The listing builds one solid part. Answer for the finished solid, in the listing's coordinates (mm). A direction names the side the tool comes from. Give positions to 0.01 mm unless a question says otherwise; leave off trailing zeros. Loops run counter-clockwise (first coordinate to the right, second up) from the corner with the lowest first, then second, coordinate; pieces in that order, holes last. Notation, with made-up numbers: M 82,68.5 L 124,68.5 A29 cw 124,88.5 Z; hole C 33,53 d1. An arc over 180 degrees is marked long. Use one line per item in the form item = value. Start each with the question number.
1. A straight line is drawn through the part: line 1 (X direction, y = -5.5, z = 11.5). Find the intervals that lie inside material, in ascending order. Write a range as from..to.
2. For faces 1 (the face through (0, -15, 8)), 2 (the face through (17, -15, -6)), 3 (the face through (35.5, -14.8, 0)), determine the directions among +Z, -Z, +X, -X, +Y, -Y from which every point of the face is accessible in a straight line to the end or side of a thin tool.
3. Each of these flat-tipped pins is pushed along its axis until it touches: pin 1 Ø5 at (y, z) = (-21, 6.5) entering from -X; pin 2 Ø1.1 at (x, y) = (35.5, -21) entering from +Z; pin 3 Ø6 at (y, z) = (-21.5, 13) entering from +X. Where does it stop, or does it pass through?
4. The part is cut by section A-A (y = -24.25). Write down the section's boundary in (x, z), and give its area (3 significant figures).
5. The part is cut by section B-B (z = 3.25). Write down the section's boundary in (x, y).
from build123d import *

# Parameters (mm, degrees)
F0_W     = 7
F0_H     = 17
F0_W_2   = 37
F0_H_2   = 2
F1_DEPTH = 30


# Not quite as in the source:
# - a feature names something its author has since deleted; it is built from what else it names


with BuildPart() as f1:
    # F0 (on Front) → F1 (new body)
    with BuildSketch(Plane.XZ):
        with Locations((31.5, 8.5)):
            Rectangle(F0_W, F0_H)
        with Locations((3.5, 8.5)):
            Rectangle(F0_W, F0_H)
        with Locations((17.5, 8.5)):
            Rectangle(F0_W, F0_H)
        with Locations((17.5, -3)):
            Rectangle(F0_W_2, F0_H_2)
        with Locations((10.5, 8.5)):
            Rectangle(F0_W, F0_H)
        Polygon((36, -4), (-1, -4), (-1, -6), (0, -6), (35, -6), (36, -6), align=None)
        Polygon((7, 0), (0, 0), (-1, 0), (-1, -2), (36, -2), (36, 0), (35, 0), (28, 0), (21, 0), (14, 0), align=None)
        with Locations((24.5, 8.5)):
            Rectangle(F0_W, F0_H)
    extrude(amount=F1_DEPTH)


solid = f1.part
Derived:
q1.line_1 = 0..35
q2.face_1 = +Z, -X, +Y, -Y
q2.face_2 = -Z, +X, -X, +Y, -Y
q2.face_3 = +Z, +X, +Y, -Y
q3.pin_1 = 0
q3.pin_2 = 17
q3.pin_3 = 35
q4.outline = M -1,-6 L 36,-6 L 36,0 L 35,0 L 35,17 L 0,17 L 0,0 L -1,0 Z
q4.area = 817 mm2
q5.outline = M 0,-30 L 35,-30 L 35,0 L 0,0 Z
